Part model, mm, in its own coordinate system. Face numbers are marked on the shaded views. A direction names the side the tool comes from. Give positions to 0.01 mm unless a question says otherwise; leave off trailing zeros. Order: outer loops, then holes, each group sorted by start corner. A loop starts at its lowest first (then second) coordinate and runs counter-clockwise, first axis right, second up. Notation, with made-up numbers: M -14,8.25 L 33,8.25 A9 cw 33,20.25 Z; hole C -17.5,-29 d10. An arc over 180 degrees is marked long. Return JSON: item names as keys, results as strings.
from build123d import *

# Parameters (mm, degrees)
SKETCH_3_R      = 1
EXTRUDE_2_DEPTH = 3
SKETCH_5_W      = 100.3
SKETCH_5_H      = 20.8
EXTRUDE_4_DEPTH = 2.5


with BuildPart() as part:
    # Sketch 3 → Extrude 2 (new body)
    with BuildSketch(Plane(origin=(0, 0, -47.45), x_dir=(-1, 0, 0), z_dir=(0, 0, -1))):
        with BuildLine():
            ThreePointArc((-20.85, 0), (-17.803910524, 7.353910524), (-10.45, 10.4))
            Line((-10.45, 10.4), (-20.85, 10.4))
            Line((-20.85, 10.4), (-32.45, 10.4))
            Line((-32.45, 10.4), (-32.45, 0))
            Line((-32.45, 0), (-20.85, 0))
        make_face()
        with BuildLine():
            Line((-20.85, -10.4), (-10.45, -10.4))
            ThreePointArc((-10.45, -10.4), (-17.803910524, -7.353910524), (-20.85, 0))
            Line((-20.85, 0), (-32.45, 0))
            Line((-32.45, 0), (-32.45, -10.4))
            Line((-32.45, -10.4), (-20.85, -10.4))
        make_face()
        with BuildLine():
            Line((-16.75, 0), (-15.45, 0))
            Line((-15.45, 0), (-15.45, 4.2))
            Line((-15.45, 4.2), (-4.45, 4.2))
            Line((-4.45, 4.2), (-4.45, 8.494704233))
            ThreePointArc((-4.45, 8.494704233), (-7.302375818, 9.912237992), (-10.45, 10.4))
            ThreePointArc((-10.45, 10.4), (-17.803910524, 7.353910524), (-20.85, 0))
            Line((-20.85, 0), (-18.75, 0))
            ThreePointArc((-18.75, 0), (-17.75, 1), (-16.75, 0))
        make_face()
        with Locations((-17.75, 3.6)):
            Circle(SKETCH_3_R, mode=Mode.SUBTRACT)
        with Locations((-14.05, 7.3)):
            Circle(SKETCH_3_R, mode=Mode.SUBTRACT)
        with Locations((-10.45, 7.3)):
            Circle(SKETCH_3_R, mode=Mode.SUBTRACT)
        with Locations((-6.85, 7.3)):
            Circle(SKETCH_3_R, mode=Mode.SUBTRACT)
        with BuildLine():
            Line((-15.45, -4.2), (-15.45, 0))
            Line((-15.45, 0), (-16.75, 0))
            ThreePointArc((-16.75, 0), (-17.75, -1), (-18.75, 0))
            Line((-18.75, 0), (-20.85, 0))
            ThreePointArc((-20.85, 0), (-17.803910524, -7.353910524), (-10.45, -10.4))
            ThreePointArc((-10.45, -10.4), (-7.302375818, -9.912237992), (-4.45, -8.494704233))
            Line((-4.45, -8.494704233), (-4.45, -4.2))
            Line((-4.45, -4.2), (-15.45, -4.2))
        make_face()
        with Locations((-17.75, -3.6)):
            Circle(SKETCH_3_R, mode=Mode.SUBTRACT)
        with Locations((-14.05, -7.3)):
            Circle(SKETCH_3_R, mode=Mode.SUBTRACT)
        with Locations((-10.45, -7.3)):
            Circle(SKETCH_3_R, mode=Mode.SUBTRACT)
        with Locations((-6.85, -7.3)):
            Circle(SKETCH_3_R, mode=Mode.SUBTRACT)
        with BuildLine():
            ThreePointArc((-10.45, 10.4), (-7.302375818, 9.912237992), (-4.45, 8.494704233))
            Line((-4.45, 8.494704233), (-4.45, 10.4))
            Line((-4.45, 10.4), (-10.45, 10.4))
        make_face()
        with BuildLine():
            Line((-4.45, -10.4), (-4.45, -8.494704233))
            ThreePointArc((-4.45, -8.494704233), (-7.302375818, -9.912237992), (-10.45, -10.4))
            Line((-10.45, -10.4), (-4.45, -10.4))
        make_face()
    extrude(amount=EXTRUDE_2_DEPTH)


with BuildPart() as body_2:
    # Mirror 7: mirrored copy
    add(part.part.mirror(Plane(origin=(0, 0, -0.3), x_dir=(1, 0, 0), z_dir=(0, 0, -1))))


with BuildPart() as part_1:
    add(part.part)

    add(body_2.part)  # Extrude 4 merges body 2
    # Sketch 5 → Extrude 4 (add)
    with BuildSketch(Plane(origin=(32.45, 0, 0), x_dir=(0, 0, -1), z_dir=(1, 0, 0))):
        with Locations((0.3, 0)):
            Rectangle(SKETCH_5_W, SKETCH_5_H)
    extrude(amount=EXTRUDE_4_DEPTH)


solid = part_1.part
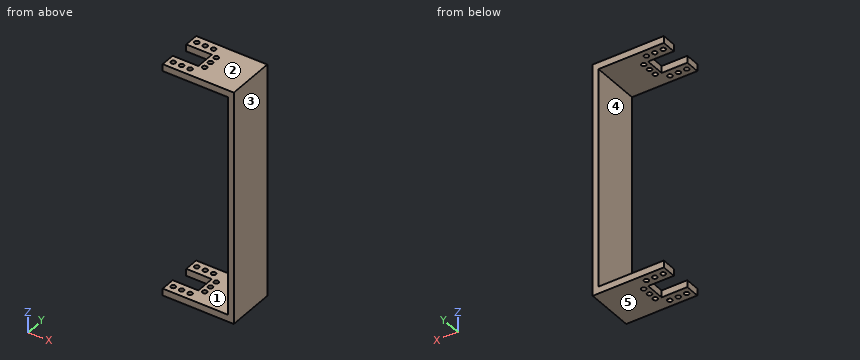
Q1. Pin check, flat tip, straight feed: pin 1 (12 mm diameter, centred on y = 6.5, z = 10, fed in from -X). Stop position of the tip, or through.
Established:
{"pin 1": "stops at x = 32.45"}
Q2. 3-axis set-ups, long thin cutter, end or side, ignore diameter. For the marked faces 4 and 5: which of +Z, -Z, +X, -X, +Y, -Y reach the whole face in a straight line?
Established:
{"face 4": "-X, +Y, -Y", "face 5": "-Z, +X, -X, +Y, -Y"}
Q3. Probe line 1 along Y through (x, z) = (10.45, 48.15); line 2 along X through (y, z) = (0, -49.8); line 3 along Z through (x, y) = (6, 8.25). List the from-to ranges inside material, lowest first.
Established:
{"line 1": "y = -10.4 to -8.3, -6.3 to -4.2, 4.2 to 6.3, 8.3 to 10.4", "line 2": "x = 15.45 to 16.75, 18.75 to 34.95", "line 3": "z = -50.45 to -47.45, 46.85 to 49.85"}
Q4. Band-saw the part on C-C (y = 0). Give the cut face in (x, z).
Established:
{"outline": "M 15.45,-50.45 L 16.75,-50.45 L 16.75,-47.45 L 15.45,-47.45 Z; M 15.45,46.85 L 16.75,46.85 L 16.75,49.85 L 15.45,49.85 Z; M 18.75,-50.45 L 34.95,-50.45 L 34.95,49.85 L 18.75,49.85 L 18.75,46.85 L 32.45,46.85 L 32.45,-47.45 L 18.75,-47.45 Z"}
Q5. Two-plate mould, pull along Z, no slides. Class the marked faces 1, 2 and 3: +Z half, -Z half, draft (parallel to the pull), parting line (faces both ways), or undercut.
Established:
{"face 1": "undercut", "face 2": "+Z half", "face 3": "draft"}
Q6. Band-saw the part on D-D (x = 22). Give the cut face in (y, z), then the cut area to 3 significant figures.
Established:
{"outline": "M -10.4,-50.45 L 10.4,-50.45 L 10.4,-47.45 L -10.4,-47.45 Z; M -10.4,46.85 L 10.4,46.85 L 10.4,49.85 L -10.4,49.85 Z", "area": "125 mm²"}
Q7. Band-saw the part on A-A (y = -7.3). Give the number of separate pieces and of enclosed holes in the cut face, then the cut area to 3 significant figures.
Established:
{"separate pieces": "7", "enclosed holes": "0", "area": "383 mm²"}
